Could you check a few things on this drawing? It's one solid part, dimensions in mm from its lowest x, y, z. A direction names the side the tool comes from. Give positions to 0.01 mm unless a question says otherwise; leave off trailing zeros. Write each loop counter-clockwise with the first axis right and the second up, starting at its lowest first coordinate (ties: lowest second). Pieces come first, ordered by that corner, then holes. Notation, with made-up numbers: M 44.5,26.5 L 59.5,26.5 A28 cw 59.5,56.5 Z; hole C -15,12 d8. An arc over 180 degrees is marked long. Answer as CSV lines item,"result". Start each with the question number.
Q1. Suppose I cut it at B-B (z = 4). Write out the boundary of the cut face in (x, y) (1 decimal).
Q2. For pin 1 (2 mm diameter, centred on y = 9.5, z = 11.5, fed in from -X) (1 decimal); pin 2 (1.5 mm diameter, centred on y = 2, z = 1.5, fed in from -X); pin 3 (5 mm diameter, centred on x = 12.7, z = 4.76, fed in from +Y) (1 decimal), each with a flat end and sliding along its axis, tell me the tip position at first contact or that it passes through.
Q3. On a 3-axis mill with a long thin cutter (end or side, diameter ignored), from which of +Z, -Z, +X, -X, +Y, -Y can I reach the whole of each face in a straight line? I mean the marked faces 1, 2 and 3. Say none if no direction works.
Q4. Suppose I cut it at C-C (x = 35). Write out the boundary of the cut face in (y, z) (1 decimal).
Q5. Suppose I cut it at A-A (x = 25.4). Write out the boundary of the cut face in (y, z) (1 decimal).
Q6. If I drill on line 1 along Y through (x, z) = (13, 9.5) (1 decimal); line 2 along Y through (x, z) = (31.75, 11.9); line 3 along X through (y, z) = (9, 12) (1 decimal), over which ranges is the centre line in solid material (lowest first)?
Q7. Suppose I cut it at D-D (z = 1.25). Write out the boundary of the cut face in (x, y) (1 decimal).
Q8. Thinking about a two-plate mould opening in Z: for the marked faces 4, 5 and 6, which applies, +Z half, -Z half, draft (parallel to the pull), parting line (faces both ways), or undercut?
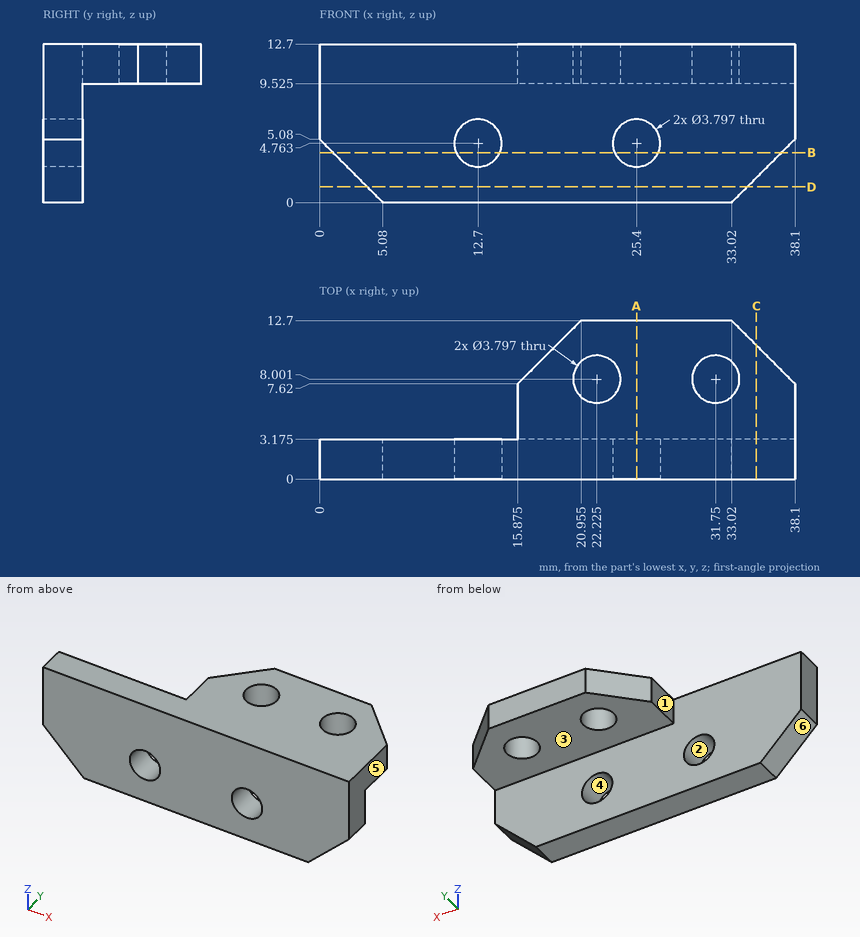
Resolved:
1,outline,"M 1.1,0 L 11,0 L 11,3.2 L 1.1,3.2 Z; M 14.4,0 L 23.7,0 L 23.7,3.2 L 14.4,3.2 Z; M 27.1,0 L 37,0 L 37,3.2 L 27.1,3.2 Z"
2,pin 1,"x = 16.8"
2,pin 2,"x = 2.83"
2,pin 3,"y = 3.2"
3,face 1,"+Z, -Z, -X, +Y"
3,face 2,"+Y, -Y"
3,face 3,"-Z, +X, -X, +Y"
4,outline,"M 0,2 L 3.2,2 L 3.2,9.5 L 10.7,9.5 L 10.7,12.7 L 0,12.7 Z"
5,outline,"M 0,0 L 3.2,0 L 3.2,2.9 L 0,2.9 Z; M 0,6.7 L 3.2,6.7 L 3.2,9.5 L 12.7,9.5 L 12.7,12.7 L 0,12.7 Z"
6,line 1,"0 to 3.2"
6,line 2,"0 to 6.1, 9.9 to 12.7"
6,line 3,"17.3 to 20.6, 23.8 to 30.1, 33.4 to 36.7"
7,outline,"M 3.8,0 L 34.3,0 L 34.3,3.2 L 3.8,3.2 Z"
8,face 4,"undercut"
8,face 5,"draft"
8,face 6,"-Z half"
